Build history of the part. All positions in model axes, mm. Give positions to 0.01 mm unless a question says otherwise; leave off trailing zeros. Order: outer loops, then holes, each group sorted by start corner. A loop starts at its lowest first (then second) coordinate and runs counter-clockwise, first axis right, second up. Notation, with made-up numbers: (17, 25.5) - (23, 25.5) arc R15 cw to (23, 51.5) - close; hole circle Ø8 at (50.5, -31). An arc over 180 degrees is marked (long way). Use a Markdown table: item, result. Add a question column.
(1) Flat gauge pins, fed straight in: pin 1 (1 mm diameter, centred on y = 1, z = -199.5, fed in from -X); pin 2 (1.5 mm diameter, centred on y = 0, z = -419.5, fed in from +X). Where does each tip first touch, or does it go through?
(2) Wall check: line 1 (Y direction, x = -6.5, z = -415.5); line 2 (X direction, y = -6.25, z = -343); line 3 (Y direction, x = 1.75, z = -154). Give the ranges that are in metal, low to high.
(3) Slice it at A-A (z = -237). Write the cut outline in (x, y), then the cut area to 3 significant figures.
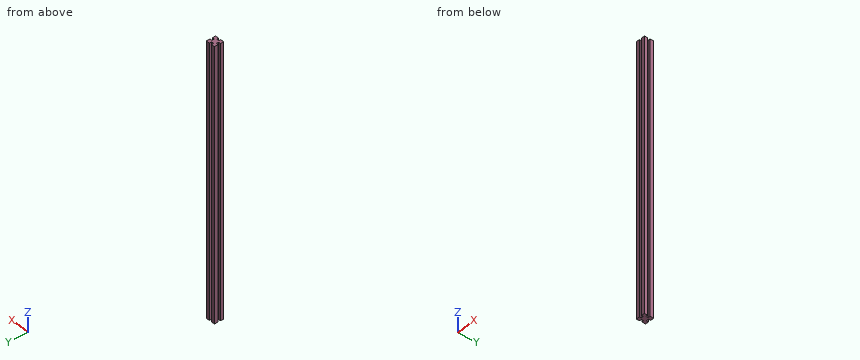
from build123d import *

# Parameters (mm, degrees)
SKETCH1_W           = 20
SKETCH1_H           = 20
BOSS_EXTRUDE1_DEPTH = 571
SKETCH2_W           = 5
SKETCH2_H           = 10
CUT_EXTRUDE1_DEPTH  = 572
CIRPATTERN1_COUNT   = 4


with BuildPart() as part:
    # Sketch1 → Boss-Extrude1 (new body)
    with BuildSketch(Plane.XY):
        Rectangle(SKETCH1_W, SKETCH1_H)
    extrude(amount=-BOSS_EXTRUDE1_DEPTH)

    # Sketch2 → Cut-Extrude1 (cut, through all)
    with BuildSketch(Plane.XY):
        with Locations((0, 10)):
            Rectangle(SKETCH2_W, SKETCH2_H)
    cut_extrude1 = extrude(amount=-CUT_EXTRUDE1_DEPTH, mode=Mode.SUBTRACT)

    # CirPattern1: Cut-Extrude1 ×4 about axis
    cirpattern1_axis = Axis((0, -0.5, 0), (0, 0, 1))
    for i in range(1, CIRPATTERN1_COUNT):
        add(cut_extrude1.rotate(cirpattern1_axis, i * 360 / CIRPATTERN1_COUNT), mode=Mode.SUBTRACT)


solid = part.part
Solution:
| question | item | result |
|---|---|---|
| 1 | pin 1 | x = -5.5 |
| 1 | pin 2 | x = 5.5 |
| 2 | line 1 | -10 to -3, 2 to 10 |
| 2 | line 2 | -10 to -2.5, 2.5 to 10 |
| 2 | line 3 | -6 to 5 |
| 3 | outline | (-10, -10) - (-2.5, -10) - (-2.5, -6) - (2.5, -6) - (2.5, -10) - (10, -10) - (10, -3) - (5.5, -3) - (5.5, 2) - (10, 2) - (10, 10) - (2.5, 10) - (2.5, 5) - (-2.5, 5) - (-2.5, 10) - (-10, 10) - (-10, 2) - (-5.5, 2) - (-5.5, -3) - (-10, -3) - close |
| 3 | area | 310 mm2 |
